from build123d import *

# Parameters (mm, degrees)
SKETCH1_R           = 2.54
BOSS_EXTRUDE1_DEPTH = 57.15
SKETCH2_R           = 0.9525
CUT_EXTRUDE1_DEPTH  = 1.905
SCALE1_SCALE        = 1.5


with BuildPart() as part:
    # Sketch1 → Boss-Extrude1 (new body)
    with BuildSketch(Plane(origin=(0, 0, 0), x_dir=(1, 0, 0), z_dir=(0, 1, 0))):
        with Locations(Location((0, 0, 0), (0, 0, 270))):
            Circle(SKETCH1_R)
    extrude(amount=BOSS_EXTRUDE1_DEPTH)

    # Sketch2 → Cut-Extrude1 (cut)
    with BuildSketch(Plane.XY.offset(2.54)):
        with Locations((0, 18.415)):
            Circle(SKETCH2_R)
        with Locations((0, 13.335)):
            Circle(SKETCH2_R)
        with Locations((0, 8.255)):
            Circle(SKETCH2_R)
        with Locations((0, 23.495)):
            Circle(SKETCH2_R)
        with Locations((0, 3.175)):
            Circle(SKETCH2_R)
    extrude(amount=-CUT_EXTRUDE1_DEPTH, mode=Mode.SUBTRACT)


with BuildPart() as part_1:
    # Scale1: scaled about (3.3e-08, 28.93183337, -0.036650166)
    add(part.part.scale(SCALE1_SCALE).moved(Location((-1.6e-08, -14.465916685, 0.018325083))))


solid = part_1.part
Geometry: final body of the model. Coordinates: model frame, mm. A direction names the side the tool comes from. Give positions to 0.01 mm unless a question says otherwise; leave off trailing zeros. Loops run counter-clockwise (first coordinate to the right, second up) from the corner with the lowest first, then second, coordinate; pieces in that order, holes last. Notation, with made-up numbers: (-26.5, 15) - (23.5, 15) arc R11 cw to (23.5, 27) - close; hole circle Ø5 at (8.25, 36). An arc over 180 degrees is marked (long way). Answer as CSV lines item,"result". Start each with the question number.
1. Ray query, L1, parallel to Y at x = 0, z = 1.95; L2, parallel to Z at x = -0.25, y = 38.5; L3, parallel to Z at x = 2.5, y = 58. Return the intervals inside material, ascending.
2. Section B-B, the plane y = 36.5. Return loops of the section in (x, z).
3. Reachability of faces 4 (the face through (0, 21, 0.971)), 5 (the face through (0, 71.259, 0)) from +Z, -Z, +X, -X, +Y, -Y: full face, straight path, thin tool, end or side. Return the list, or none.
4. Pin query (flat end, axial travel): P1, Ø0.9, axis at x = 0, y = 13, coming from the +Z side; P2, Ø1, axis at y = 45, z = -1.5, coming from the +X side; P3, Ø2, axis at x = -1.5, y = 59, coming from the +Z side. Return the tip coordinate at first contact, or that it passes through.
5. Section C-C, the plane z = -2.75. Return loops of the section in (x, y).
6. Draft query along X for faces 1 (the face through (1.36, 21.21, 2.42)), 2 (the face through (0.168, 27.797, -3.788)), 3 (the face through (0, -14.466, 0)). Return one class per face: released by +X, released by -X, zero draft, split by the parting line, or undercut.
7. Section A-A, the plane x = 0. Return loops of the section in (y, z).
Answers:
1,L1,"y = -14.47 to -11.13, -8.27 to -3.51, -0.65 to 4.11, 6.97 to 11.73, 14.59 to 19.35, 22.21 to 71.26"
1,L2,"z = -3.78 to 3.82"
1,L3,"z = -2.86 to 2.89"
2,outline,"circle Ø7.62 at (0, 0.02)"
3,face 4,"+Z"
3,face 5,"+Z, -Z, +X, -X, +Y"
4,P1,"stops at z = 0.97"
4,P2,"stops at x = 3.67"
4,P3,"stops at z = 3.8"
5,outline,"(-2.62, -14.47) - (2.62, -14.47) - (2.62, 71.26) - (-2.62, 71.26) - close"
6,face 1,"undercut"
6,face 2,"split by the parting line"
6,face 3,"zero draft"
7,outline,"(-14.47, -3.79) - (71.26, -3.79) - (71.26, 3.83) - (22.21, 3.83) - (22.21, 0.97) - (19.35, 0.97) - (19.35, 3.83) - (14.59, 3.83) - (14.59, 0.97) - (11.73, 0.97) - (11.73, 3.83) - (6.97, 3.83) - (6.97, 0.97) - (4.11, 0.97) - (4.11, 3.83) - (-0.65, 3.83) - (-0.65, 0.97) - (-3.51, 0.97) - (-3.51, 3.83) - (-8.27, 3.83) - (-8.27, 0.97) - (-11.13, 0.97) - (-11.13, 3.83) - (-14.47, 3.83) - close"
